```python
from build123d import *

# Parameters (mm, degrees)
ESTRUSIONE_ESTRUSIONE1_DEPTH = 33
RACCORDO1_R                  = 1
SCHIZZO2_R                   = 6
TAGLIO_ESTRUSIONE1_DEPTH     = 5
SCHIZZO3_R                   = 4.46
TAGLIO_ESTRUSIONE2_DEPTH     = 2
SCHIZZO4_R                   = 2.65
TAGLIO_ESTRUSIONE3_DEPTH     = 8
SCHIZZO5_R                   = 2
ESTRUSIONE_ESTRUSIONE2_DEPTH = 5


with BuildPart() as part:
    # Schizzo1 → Estrusione-Estrusione1 (new body)
    with BuildSketch(Plane.XY):
        with BuildLine():
            Line((-75.5, -15), (75.5, -15))
            ThreePointArc((75.5, -15), (87.5, 0), (75.5, 15))
            Line((75.5, 15), (-75.5, 15))
            ThreePointArc((-75.5, 15), (-87.5, 0), (-75.5, -15))
        make_face()
    extrude(amount=ESTRUSIONE_ESTRUSIONE1_DEPTH)

    # Raccordo1
    # the kernel refuses this fillet: 1 mm, written as the material it takes off along each edge
    with BuildSketch(Plane(origin=(72.125, 0, 33), x_dir=(0.05848647839975847, -0.9982882007939364, 0), z_dir=(-0.9982882007939364, -0.05848647839975847, 0))) as raccordo1_piece_1:
        with BuildLine():
            CenterArc((15.375 - RACCORDO1_R, -RACCORDO1_R), RACCORDO1_R, 0, 90)
            Line((15.375 - RACCORDO1_R, 0), (15.375, 0))
            Line((15.375, 0), (15.375, -RACCORDO1_R))
        make_face()
    revolve(axis=Axis((72.125, 0, 33), (0, 0, 1)), revolution_arc=173.294116446, mode=Mode.SUBTRACT)
    with BuildSketch(Plane(origin=(78, 15, 33), x_dir=(0, 0, -1), z_dir=(-1, 0, 0)), Plane(origin=(-78, -15, 33), x_dir=(0, 0, -1), z_dir=(1, 0, 0))) as raccordo1_piece_2:
        with BuildLine():
            CenterArc((RACCORDO1_R, RACCORDO1_R), RACCORDO1_R, 180, 90)
            Line((0, RACCORDO1_R), (0, 0))
            Line((0, 0), (RACCORDO1_R, 0))
        make_face()
    extrude(amount=156, mode=Mode.SUBTRACT)
    with BuildSketch(Plane(origin=(-72.125, 0, 33), x_dir=(-0.05848647839975752, 0.9982882007939364, 0), z_dir=(0.9982882007939364, 0.05848647839975752, 0))) as raccordo1_piece_3:
        with BuildLine():
            CenterArc((15.375 - RACCORDO1_R, -RACCORDO1_R), RACCORDO1_R, 0, 90)
            Line((15.375 - RACCORDO1_R, 0), (15.375, 0))
            Line((15.375, 0), (15.375, -RACCORDO1_R))
        make_face()
    revolve(axis=Axis((-72.125, 0, 33), (0, 0, 1)), revolution_arc=173.294116446, mode=Mode.SUBTRACT)

    # Schizzo2 → Taglio-Estrusione1 (cut)
    with BuildSketch(Plane.XY.offset(33)):
        with Locations((-60, 0)):
            Circle(SCHIZZO2_R)
        with Locations((60, 0)):
            Circle(SCHIZZO2_R)
    extrude(amount=-TAGLIO_ESTRUSIONE1_DEPTH, mode=Mode.SUBTRACT)

    # Schizzo3 → Taglio-Estrusione2 (cut)
    with BuildSketch(Plane.XZ.offset(15)):
        with Locations((0, 15.6)):
            Circle(SCHIZZO3_R)
    extrude(amount=-TAGLIO_ESTRUSIONE2_DEPTH, mode=Mode.SUBTRACT)

    # Schizzo4 → Taglio-Estrusione3 (cut)
    with BuildSketch(Plane.XZ.offset(13)):
        with Locations((0, 15.6)):
            Circle(SCHIZZO4_R)
    extrude(amount=-TAGLIO_ESTRUSIONE3_DEPTH, mode=Mode.SUBTRACT)

    # Schizzo5 → Estrusione-Estrusione2 (add)
    with BuildSketch(Plane(origin=(0, 0, 0), x_dir=(-1, 0, 0), z_dir=(0, 0, -1))):
        with Locations(Location((0, -10, 0), (0, 0, 180))):
            Circle(SCHIZZO5_R)
    extrude(amount=ESTRUSIONE_ESTRUSIONE2_DEPTH)


solid = part.part
```
Part model, mm, in its own coordinate system. A direction names the side the tool comes from. Round coordinates to 2 decimals unless told otherwise and drop trailing zeros. Write each loop counter-clockwise with the first axis right and the second up, starting at its lowest first coordinate (ties: lowest second). Pieces come first, ordered by that corner, then holes.
Item 1: Cut at A-A, the plane z = 30.5. Give the cut face in (x, y) (3 decimals).
Results:
outline: (-75.5, -15) - (75.5, -15) arc R15.375 ccw to (75.5, 15) - (-75.5, 15) arc R15.375 ccw to start; hole circle Ø12 at (-60, 0); hole circle Ø12 at (60, 0)
Item 2: Probe L1, parallel to Z at x = 0, y = -7; L2, parallel to Y at x = 60, z = 31.95; L3, parallel to Z at x = 56, y = 8.5. List the from-to ranges inside material, lowest first.
Results:
L1: z = 0 to 12.95, 18.25 to 33
L2: y = -15 to -6, 6 to 15
L3: z = 0 to 33
Item 3: Cut at D-D, the plane x = 60. Give the cut face in (y, z).
Results:
outline: (-15, 0) - (15, 0) - (15, 32) arc R1 ccw to (14, 33) - (6, 33) - (6, 28) - (-6, 28) - (-6, 33) - (-14, 33) arc R1 ccw to (-15, 32) - close
Item 4: Drop flat-ended pins along their axis: pin 1 Ø3 at (x, y) = (27, 9.5) entering from -Z; pin 2 Ø4.5 at (x, z) = (0.5, 15.5) entering from -Y; pin 3 Ø3.5 at (x, y) = (-60, 0.5) entering from +Z. Give the stop position or say it passes through.
Results:
pin 1: stops at z = 0
pin 2: stops at y = -13
pin 3: stops at z = 28
Item 5: Two-plate mould, pull along Y, no slides. Class faces 1 (the cylindrical face through (-87.497, 0.29, 15.776)), 2 (the flat face through (60, 0, 28)), 3 (the flat face through (-1, -15, 9)): +Y half, -Y half, draft (parallel to the pull), parting line (faces both ways), or undercut.
Results:
face 1: parting line
face 2: undercut
face 3: -Y half
Item 6: Cut at B-B, the plane x = 0. Give the cut face in (y, z), plus the area to 3 significant figures.
Results:
outline: (-15, 0) - (-12, 0) - (-12, -5) - (-8, -5) - (-8, 0) - (15, 0) - (15, 32) arc R1 ccw to (14, 33) - (-14, 33) arc R1 ccw to (-15, 32) - (-15, 20.06) - (-13, 20.06) - (-13, 18.25) - (-5, 18.25) - (-5, 12.95) - (-13, 12.95) - (-13, 11.14) - (-15, 11.14) - close
area: 949 mm2
Item 7: Cut at C-C, the plane y = 0. Give the cut face in (x, z).
Results:
outline: (-87.5, 0) - (87.5, 0) - (87.5, 32) arc R1 ccw to (86.5, 33) - (66, 33) - (66, 28) - (54, 28) - (54, 33) - (-54, 33) - (-54, 28) - (-66, 28) - (-66, 33) - (-86.5, 33) arc R1 ccw to (-87.5, 32) - close
Item 8: Which spindle directions (+Z, -Z, +X, -X, +Y, -Y) get a long thin tool onto all of the face, cutting with end or side? Do faces 4 (the flat face through (-1, 0, 33)), 5 (the cylindrical face through (2.528, -9.056, 16.396)), 6 (the cylindrical face through (-66, 0, 31)), 7 (the cylindrical face through (0, -12, -2)). Say none if no direction does.
Results:
face 4: +Z, +X, -X, +Y, -Y
face 5: -Y
face 6: +Z
face 7: -Z
